from build123d import *

# Parameters (mm, degrees)
BOSS_EXTRUDE1_DEPTH = 6
SKETCH2_W           = 1
SKETCH2_H           = 15
CUT_EXTRUDE1_DEPTH  = 190.977931876


with BuildPart() as part:
    # Sketch1 → Boss-Extrude1 (new body)
    with BuildSketch(Plane(origin=(0, 0, 0), x_dir=(1, 0, 0), z_dir=(0, 1, 0))):
        with BuildLine():
            Line((0, 7.11), (182.64, 7.11))
            ThreePointArc((182.64, 7.11), (189.75, 0), (182.64, -7.11))
            Line((182.64, -7.11), (0, -7.11))
            ThreePointArc((0, -7.11), (-7.11, 0), (0, 7.11))
        make_face()
        with BuildLine():
            Line((0, 6.112197724), (182.64, 6.112197724))
            ThreePointArc((182.64, 6.112197724), (188.752197724, 0), (182.64, -6.112197724))
            Line((182.64, -6.112197724), (0, -6.112197724))
            ThreePointArc((0, -6.112197724), (-6.112197724, 0), (0, 6.112197724))
        make_face(mode=Mode.SUBTRACT)
    extrude(amount=BOSS_EXTRUDE1_DEPTH)

    # Sketch2 → Cut-Extrude1 (cut, through all)
    with BuildSketch(Plane(origin=(0, 6, 0), x_dir=(1, 0, 0), z_dir=(0, 1, 0))):
        with Locations((189.75, 0)):
            Rectangle(SKETCH2_W, SKETCH2_H)
        with Locations((-7.11, 0)):
            Rectangle(SKETCH2_W, SKETCH2_H)
    extrude(amount=-CUT_EXTRUDE1_DEPTH, mode=Mode.SUBTRACT)


solid = part.part
Input: part model. Units: mm. Frame: model coordinates. A direction names the side the tool comes from. Round coordinates to 2 decimals unless told otherwise and drop trailing zeros. Order: outer loops, then holes, each group sorted by start corner. A loop starts at its lowest first (then second) coordinate and runs counter-clockwise, first axis right, second up.
1. Mould query, pull axis X, two halves, no side actions, for faces 1 (the face through (91.8, 0, -6.4)), 2 (the face through (186.68, 2.96, 5.85)), 3 (the face through (-6.11, 2.96, 0.13)), 4 (the face through (188.75, 2.96, -0.13)). Classes: released by +X, released by -X, zero draft, split by the parting line, or undercut.
The answers:
face 1: zero draft
face 2: released by +X
face 3: undercut
face 4: undercut
2. Material intervals for line 1 (Z direction, x = 100, y = 4.15); line 2 (X direction, y = 0.3, z = -0.5), sorted ascending.
The answers:
line 1: z = -7.11 to -6.11, 6.11 to 7.11
line 2: x = -6.61 to -6.09, 188.73 to 189.25
3. Cut plane C-C, the plane x = 29. Output: boundary loops of the cut face in (y, z).
The answers:
outline: (0, -7.11) - (6, -7.11) - (6, -6.11) - (0, -6.11) - close; (0, 6.11) - (6, 6.11) - (6, 7.11) - (0, 7.11) - close
4. Set-up query: faces 5 (the face through (90, 3, -6.112)), 6 (the face through (189.25, 3, 0)). Return all of +Z, -Z, +X, -X, +Y, -Y with unobstructed straight access to the full face (end or side cutting, diameter ignored); none if empty.
The answers:
face 5: +Y, -Y
face 6: +Z, -Z, +X, +Y, -Y
5. Cut plane A-A, the plane z = 0. Output: boundary loops of the cut face in (x, y), then the cut area to 3 significant figures.
The answers:
outline: (-6.61, 0) - (-6.11, 0) - (-6.11, 6) - (-6.61, 6) - close; (188.75, 0) - (189.25, 0) - (189.25, 6) - (188.75, 6) - close
area: 5.97 mm2
6. Cut plane B-B, the plane y = 2.3. Output: boundary loops of the cut face in (x, z), then the cut area to 3 significant figures.
The answers:
outline: (-6.61, -2.62) arc R7.11 ccw to (0, -7.11) - (182.64, -7.11) arc R7.11 ccw to (189.25, -2.62) - (189.25, 2.62) arc R7.11 ccw to (182.64, 7.11) - (0, 7.11) arc R7.11 ccw to (-6.61, 2.62) - close; hole (0, -6.11) - (182.64, -6.11) arc R6.11 ccw to (182.64, 6.11) - (0, 6.11) arc R6.11 ccw to start
area: 402 mm2
